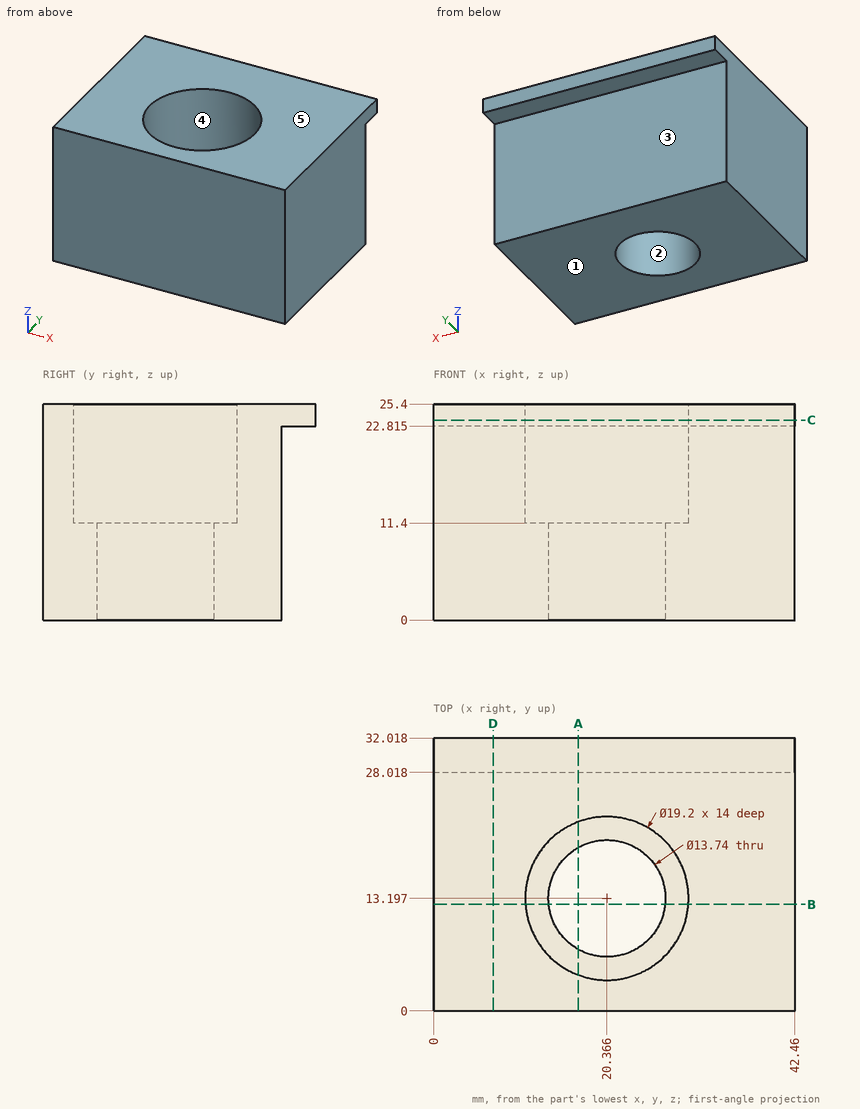
Input: dimensioned drawing with shaded views. Units: mm. Origin: part minimum x, y, z. A direction names the side the tool comes from. Round coordinates to 2 decimals unless told otherwise and drop trailing zeros. Loops run counter-clockwise (first coordinate to the right, second up) from the corner with the lowest first, then second, coordinate; pieces in that order, holes last. Notation, with made-up numbers: (-10, 87.5) -> (39, 87.5) arc R21 cw to (39, 125.5) -> close; hole circle Ø11 at (4, 3.5). An arc over 180 degrees is marked (long way). Answer as a JSON object with one key per item and string values. Group by question number.
1) Section query C-C on z = 23.5. Output: boundary loops of the cut face in (x, y), plus the area to 3 significant figures.
2) Draft query along Y for the marked faces 1, 2 and 3. Return one class per face: +Y half, -Y half, draft (parallel to the pull), parting line (faces both ways), or undercut.
3) Section query D-D on x = 7. Output: boundary loops of the cut face in (y, z) (1 decimal).
4) Section query B-B on y = 12.5. Output: boundary loops of the cut face in (x, z).
5) Pin query (flat end, axial travel): pin 1 (12.5 mm diameter, centred on x = 20.37, y = 13.2, fed in from +Z); pin 2 (11.5 mm diameter, centred on x = 16, z = 8.5, fed in from +Y). Return the tip coordinate at first contact, or that it passes through.
6) Ray query, L1, parallel to Y at x = 12, z = 10.25; L2, parallel to Z at x = 20, y = 22; L3, parallel to X at y = 10.5, z = 17.5. Return the intervals inside material, ascending.
7) Section query A-A on x = 17. Output: boundary loops of the cut face in (y, z) (1 decimal), plus the area to 3 significant figures.
8) Reachability of the marked faces 4 and 5 from +Z, -Z, +X, -X, +Y, -Y: full face, straight path, thin tool, end or side. Return the list, or none.
Reply:
{
 "1": {"outline": "(0, 0) -> (42.46, 0) -> (42.46, 32.02) -> (0, 32.02) -> close; hole circle Ø19.2 at (20.37, 13.2)", "area": "1,070 mm2"},
 "2": {"face 1": "draft", "face 2": "undercut", "face 3": "+Y half"},
 "3": {"outline": "(0, 0) -> (28, 0) -> (28, 22.8) -> (32, 22.8) -> (32, 25.4) -> (0, 25.4) -> close"},
 "4": {"outline": "(0, 0) -> (13.53, 0) -> (13.53, 11.4) -> (10.79, 11.4) -> (10.79, 25.4) -> (0, 25.4) -> close; (27.2, 0) -> (42.46, 0) -> (42.46, 25.4) -> (29.94, 25.4) -> (29.94, 11.4) -> (27.2, 11.4) -> close"},
 "5": {"pin 1": "passes through", "pin 2": "stops at y = 28.02"},
 "6": {"L1": "y = 0 to 28.02", "L2": "z = 0 to 11.4", "L3": "x = 0 to 11.15, 29.58 to 42.46"},
 "7": {"outline": "(0, 0) -> (7.2, 0) -> (7.2, 11.4) -> (4.2, 11.4) -> (4.2, 25.4) -> (0, 25.4) -> close; (19.2, 0) -> (28, 0) -> (28, 22.8) -> (32, 22.8) -> (32, 25.4) -> (22.2, 25.4) -> (22.2, 11.4) -> (19.2, 11.4) -> close", "area": "334 mm2"},
 "8": {"face 4": "+Z", "face 5": "+Z, +X, -X, +Y, -Y"}
}
